```python
from build123d import *

# Parameters (mm, degrees)
PAD009_DEPTH    = 1.8
SKETCH033_R     = 4
POCKET021_DEPTH = 5
SKETCH_W        = 2
SKETCH_H        = 3.3
SKETCH_W_2      = 4
PAD_DEPTH       = 20


with BuildPart() as part:
    # Sketch031 → Pad009 (new body)
    with BuildSketch(Plane.XY):
        Polygon((-13, 13.75), (13, 13.75), (13, 10.45), (9, 10.45), (9, -5.45), (13, -5.45), (13, -8.75), (-13, -8.75), (-13, -5.45), (-9, -5.45), (-9, 10.45), (-13, 10.45), align=None)
    extrude(amount=PAD009_DEPTH)

    # Sketch033 → Pocket021 (cut)
    with BuildSketch(Plane.XY.offset(2)):
        Circle(SKETCH033_R)
    extrude(amount=-POCKET021_DEPTH, mode=Mode.SUBTRACT)

    # Sketch (on Face13 of Pad009) → Pad (join)
    with BuildSketch(Plane(origin=(0, 0, 0), x_dir=(1, 0, 0), z_dir=(0, 0, -1))):
        with Locations((-12, 7.1)):
            Rectangle(SKETCH_W, SKETCH_H)
        with Locations((11, 7.1)):
            Rectangle(SKETCH_W_2, SKETCH_H)
        with Locations((11, -12.1)):
            Rectangle(SKETCH_W_2, SKETCH_H)
        with Locations((-11, -12.1)):
            Rectangle(SKETCH_W_2, SKETCH_H)
    extrude(amount=PAD_DEPTH)


with BuildPart() as part_1:
    # Body005 placement: moved
    add(part.part.moved(Location((0, 0, 28))))


solid = part_1.part
```
Read the model definition and answer for the solid it produces. Units are mm, in the model's axes. A direction names the side the tool comes from. Coordinates: 2 decimals unless noted, no trailing zeros. Write each loop counter-clockwise with the first axis right and the second up, starting at its lowest first coordinate (ties: lowest second). Pieces come first, ordered by that corner, then holes. Notation, with made-up numbers: (-13.5, -33.75) -> (39.5, -33.75) arc R10 ccw to (39.5, -15.75) -> close; hole circle Ø2 at (56, 56.25). An arc over 180 degrees is marked (long way). Write item = value, one per line.
(1) Which of the six approach directions +Z, -Z, +X, -X, +Y, -Y give full straight-line access (tool end or side, diameter ignored) to faces 5 (the face through (-9, 2, 29)), 6 (the face through (10, -8.75, 21)), 7 (the face through (9, 3, 29)), 8 (the face through (9, 12, 18))?
From the geometry:
face_5 = +Z, -Z, -X
face_6 = +Z, -Z, +X, -X, -Y
face_7 = +Z, -Z, +X
face_8 = -Z, +Y, -Y
(2) For a pull along X with two mould halves and no side action, classify faces 1 (the face through (-0.867, -3.905, 28.913)), 2 (the face through (-1, 5, 28)), 3 (the face through (-13, 12, 19)), 4 (the face through (-12, -7, 8)) as +X half, -X half, draft (parallel to the pull), parting line (faces both ways), or undercut.
From the geometry:
face_1 = undercut
face_2 = undercut
face_3 = -X half
face_4 = draft
(3) Section D-D on y = 9.75 is taken. Write down the section's boundary in (x, z), plus the area to 3 significant figures.
From the geometry:
outline = (-9, 28) -> (9, 28) -> (9, 29.8) -> (-9, 29.8) -> close
area = 32.4 mm2
(4) Straight lines are drawn through the part: L1, parallel to Y at x = 0, z = 28.55; L2, parallel to X at y = 11.75, z = 26.5; L3, parallel to Y at x = 11.75, z = 12.75. For each, find the intervals that lie inside material, in ascending order. Write a range as from..to.
From the geometry:
L1 = -8.75..-4, 4..13.75
L2 = -13..-9, 9..13
L3 = -8.75..-5.45, 10.45..13.75
(5) Section B-B on z = 22.25 is taken. Write down the section's boundary in (x, y).
From the geometry:
outline = (-13, -8.75) -> (-11, -8.75) -> (-11, -5.45) -> (-13, -5.45) -> close; (-13, 10.45) -> (-9, 10.45) -> (-9, 13.75) -> (-13, 13.75) -> close; (9, -8.75) -> (13, -8.75) -> (13, -5.45) -> (9, -5.45) -> close; (9, 10.45) -> (13, 10.45) -> (13, 13.75) -> (9, 13.75) -> close
(6) Section A-A on y = 0 is taken. Write down the section's boundary in (x, z).
From the geometry:
outline = (-9, 28) -> (-4, 28) -> (-4, 29.8) -> (-9, 29.8) -> close; (4, 28) -> (9, 28) -> (9, 29.8) -> (4, 29.8) -> close
(7) Given pin 1 Ø1.4 at (y, z) = (6, 29) entering from -X; pin 2 Ø0.9 at (y, z) = (-1, 29) entering from +X, each flat-ended and moving along its own axis, determine where each tip first touches the part or whether it passes through.
From the geometry:
pin_1 = -9
pin_2 = 9
(8) Section C-C on x = 0 is taken. Write down the section's boundary in (y, z).
From the geometry:
outline = (-8.75, 28) -> (-4, 28) -> (-4, 29.8) -> (-8.75, 29.8) -> close; (4, 28) -> (13.75, 28) -> (13.75, 29.8) -> (4, 29.8) -> close
